Geometry check sheet. Reference: the model listing, model coordinates, mm. A direction names the side the tool comes from. Coordinates: 2 decimals unless noted, no trailing zeros. Order: outer loops, then holes, each group sorted by start corner. A loop starts at its lowest first (then second) coordinate and runs counter-clockwise, first axis right, second up. Notation, with made-up numbers: (-7, 15.5) - (37, 15.5) arc R26 ccw to (37, 42.5) - close; hole circle Ø1 at (-23, 38). An arc over 180 degrees is marked (long way). Return JSON: item names as keys, results as strings. Group by question number.
Item 1: Tool access check on faces 1 (the flat face through (13, 15, -13)), 2 (the flat face through (0, 0, 0)). Record the directions out of +Z, -Z, +X, -X, +Y, -Y that give a thin tool (end or side, any length) a straight path to the whole face; none if there is none.
Item 2: Section check A-A on x = 0. Enter the section's corners in (y, z), then the cut area to 3 significant figures.
Item 3: Section check C-C on x = 9.5. Enter the section's corners in (y, z), then the cut area to 3 significant figures.
Item 4: Section check D-D on y = 112.5. Enter the section's corners in (x, z), then the cut area to 3 significant figures.
Item 5: Scan lines: probe 1 along Y at (x, z) = (0, 12.5); probe 2 along Y at (x, z) = (7, 21.5); probe 3 along Z at (x, y) = (-1, 36.5). Record each from-to range of solid material in increasing order.
Item 6: Section check B-B on z = 16. Enter the section's corners in (x, y), then the cut area to 3 significant figures.
Item 7: Gauge pin test, flat ends, axial feed: pin 1 (3 mm diameter, centred on x = -10.5, y = 97, fed in from -Z); pin 2 (1 mm diameter, centred on x = -19, y = 95.5, fed in from +Z); pin 3 (8 mm diameter, centred on x = -3.5, y = 70.5, fed in from -Z); pin 4 (6 mm diameter, centred on x = -5.5, y = 68, fed in from +Z) (3 decimals). Record the tip position at first contact, or that the pin passes through.
from build123d import *

# Parameters (mm, degrees)
SKETCH3_R               = 3.75
CUT_EXTRUDE1_DEPTH      = 31
CUT_EXTRUDE1_DEPTH_BACK = 31


with BuildPart() as part:
    # Sketch2 → Revolve1 (revolve)
    with BuildSketch(Plane.XY):
        Polygon((0, 0), (30, 0), (30, 15), (17.7222, 15), (17.7222, 125), (0, 125), align=None)
    revolve(axis=Axis((0, 125, 0), (0, -1, 0)))

    # Sketch3 → Cut-Extrude1 (cut, two sides)
    with BuildSketch(Plane.XY) as cut_extrude1_sk:
        with Locations((0, 112.5)):
            Circle(SKETCH3_R)
    extrude(amount=CUT_EXTRUDE1_DEPTH, mode=Mode.SUBTRACT)
    extrude(cut_extrude1_sk.sketch, amount=-CUT_EXTRUDE1_DEPTH_BACK, mode=Mode.SUBTRACT)


solid = part.part
Computed:
{
 "1": {"face 1": "+Y", "face 2": "+Z, -Z, +X, -X, -Y"},
 "2": {"outline": "(0, -30) - (15, -30) - (15, -17.72) - (108.75, -17.72) - (108.75, 17.72) - (15, 17.72) - (15, 30) - (0, 30) - close; (116.25, -17.72) - (125, -17.72) - (125, 17.72) - (116.25, 17.72) - close", "area": "4,530 mm²"},
 "3": {"outline": "(0, -28.46) - (15, -28.46) - (15, -14.96) - (125, -14.96) - (125, 14.96) - (15, 14.96) - (15, 28.46) - (0, 28.46) - close", "area": "4,150 mm²"},
 "4": {"outline": "(-3.75, -17.32) - (-3.75, 17.32) arc R17.72 ccw to start; (3.75, -17.32) arc R17.72 ccw to (3.75, 17.32) - close", "area": "723 mm²"},
 "5": {"probe 1": "y = 0 to 108.75, 116.25 to 125", "probe 2": "y = 0 to 15", "probe 3": "z = -17.69 to 17.69"},
 "6": {"outline": "(-25.38, 0) - (25.38, 0) - (25.38, 15) - (7.62, 15) - (7.62, 125) - (-7.62, 125) - (-7.62, 15) - (-25.38, 15) - close; hole circle Ø7.5 at (0, 112.5)", "area": "2,390 mm²"},
 "7": {"pin 1": "stops at z = -15.27", "pin 2": "passes through", "pin 3": "stops at z = -17.72", "pin 4": "stops at z = 17.545"}
}
